The figure shows three views and two pictorial views of one solid part (mm, origin at its lowest corner). Answer the questions. A direction names the side the tool comes from. Give positions to 0.01 mm unless a question says otherwise; leave off trailing zeros. Order: outer loops, then holes, each group sorted by start corner. A loop starts at its lowest first (then second) coordinate and runs counter-clockwise, first axis right, second up. Notation, with made-up numbers: (79.25, 71.25) - (90.25, 71.25) arc R21 cw to (90.25, 108.25) - close; hole circle Ø2 at (47, 74). An arc over 180 degrees is marked (long way). Return JSON: item names as keys, results as strings. Group by question number.
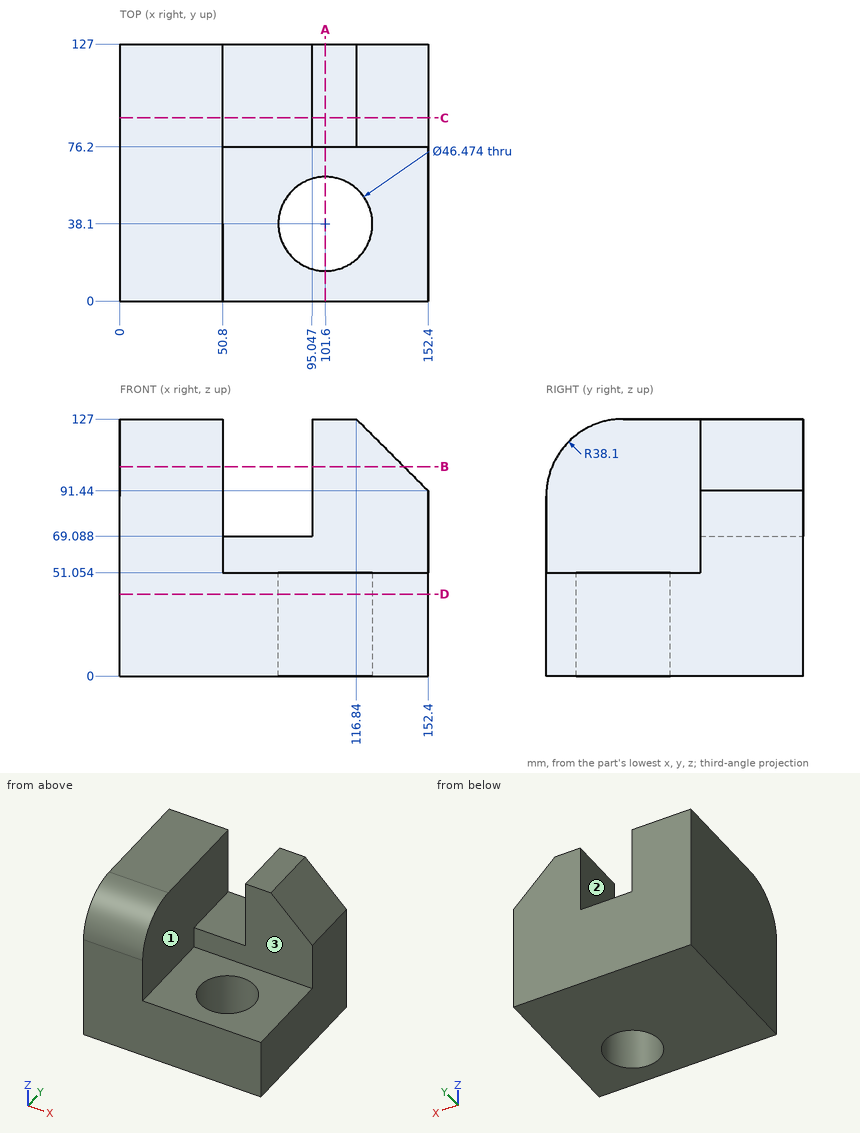
1. A tool of negligible diameter and unlimited length cuts with its end or side. For the marked faces 1, 2 and 3, from which of +Z, -Z, +X, -X, +Y, -Y can it reach the whole face along a straight path? Write none if from no direction.
2. The part is cut by section C-C (y = 90.5). Give the vertices of the cut face in (x, z), and give its area (3 significant figures).
3. The part is cut by section A-A (x = 101.6). Give the vertices of the cut face in (y, z), and give its area (3 significant figures).
4. The part is cut by section B-B (z = 103.5). Give the vertices of the cut face in (x, y).
5. Consider probe 1 along Y at (x, z) = (101, 28); probe 2 along X at (y, z) = (38.5, 50.5); probe 3 along X at (y, z) = (43, 85). Determine where each line is inside the solid, lowest interval first. Write a range as from..to.
6. The part is cut by section D-D (z = 40.5). Give the vertices of the cut face in (x, y).
7. Each of these flat-tipped pins is pushed along its axis until it touches: pin 1 (12 mm diameter, centred on x = 102, z = 88, fed in from -Y); pin 2 (3 mm diameter, centred on x = 66, y = 79.5, fed in from +Z); pin 3 (1 mm diameter, centred on y = 23.5, z = 83, fed in from +X). Where does it stop, or does it pass through?
Answers:
{
 "1": {"face 1": "+Z, -Y", "face 2": "+Z, +Y, -Y", "face 3": "+Z, +X, -Y"},
 "2": {"outline": "(0, 0) - (152.4, 0) - (152.4, 91.44) - (116.84, 127) - (95.05, 127) - (95.05, 69.09) - (50.8, 69.09) - (50.8, 127) - (0, 127) - close", "area": "16,200 mm^2"},
 "3": {"outline": "(0, 0) - (14.86, 0) - (14.86, 51.05) - (0, 51.05) - close; (61.34, 0) - (127, 0) - (127, 127) - (76.2, 127) - (76.2, 51.05) - (61.34, 51.05) - close", "area": "7,970 mm^2"},
 "4": {"outline": "(0, 2.91) - (50.8, 2.91) - (50.8, 127) - (0, 127) - close; (95.05, 76.2) - (140.34, 76.2) - (140.34, 127) - (95.05, 127) - close"},
 "5": {"probe 1": "y = 0..14.87, 61.33..127", "probe 2": "x = 0..78.37, 124.83..152.4", "probe 3": "x = 0..50.8"},
 "6": {"outline": "(0, 0) - (152.4, 0) - (152.4, 127) - (0, 127) - close; hole circle Ø46.47 at (101.6, 38.1)"},
 "7": {"pin 1": "stops at y = 76.2", "pin 2": "stops at z = 69.09", "pin 3": "stops at x = 50.8"}
}
